Can you work these out from the drawing? Everything is in mm from the part's minimum corner. Coordinates: 2 decimals unless noted, no trailing zeros. Order: outer loops, then holes, each group sorted by start corner. A loop starts at its lowest first (then second) coordinate and runs counter-clockwise, first axis right, second up. Notation, with made-up numbers: (79.25, 63.5) - (135.25, 63.5) arc R28 cw to (135.25, 97.5) - close; hole circle Ø11 at (7, 13.25). An arc over 180 degrees is marked (long way). Answer as CSV lines item,"result". Start each with the question number.
Q1. I need wall thicknesses on line 1 (X direction, y = 7.25, z = 4.75) (1 decimal); line 2 (Z direction, x = 53.5, y = 13.5) (1 decimal); line 3 (X direction, y = 8.25, z = 3.75) (1 decimal). Which ranges of each line are inside material? Lowest first, please.
Q2. Suppose I cut it at B-B (y = 4.5). Please give me the cut outline in (x, z) (1 decimal).
Q3. For pin 1 Ø1 at (x, y) = (29, 3) entering from -Z, with a flat end and sliding along its axis, tell me the tip position at first contact or that it passes through.
Q4. Thinking about a two-plate mould opening in X: for the marked faces 1, 2 and 3, which applies, released by +X, released by -X, zero draft, split by the parting line, or undercut?
Q5. Suppose I cut it at A-A (x = 53.5). Please give me the cut outline in (y, z) (1 decimal), then the cut area to 3 significant figures.
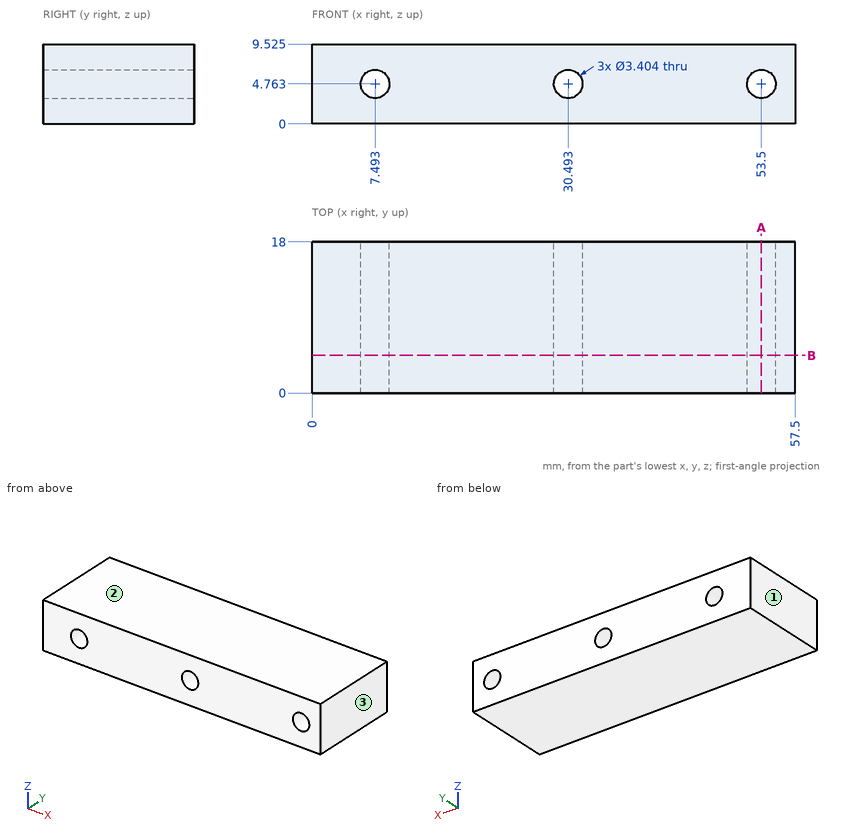
Here are the results:
1,line 1,"x = 0 to 5.8, 9.2 to 28.8, 32.2 to 51.8, 55.2 to 57.5"
1,line 2,"z = 0 to 3.1, 6.5 to 9.5"
1,line 3,"x = 0 to 6.1, 8.9 to 29.1, 31.9 to 52.1, 54.9 to 57.5"
2,outline,"(0, 0) - (57.5, 0) - (57.5, 9.5) - (0, 9.5) - close; hole circle Ø3.4 at (7.5, 4.8); hole circle Ø3.4 at (30.5, 4.8); hole circle Ø3.4 at (53.5, 4.8)"
3,pin 1,"stops at z = 0"
4,face 1,"released by -X"
4,face 2,"zero draft"
4,face 3,"released by +X"
5,outline,"(0, 0) - (18, 0) - (18, 3.1) - (0, 3.1) - close; (0, 6.5) - (18, 6.5) - (18, 9.5) - (0, 9.5) - close"
5,area,"110 mm²"
